```python
from build123d import *

# Parameters (mm, degrees)
F3_DEPTH  = 7.001
F4_W      = 1.95
F4_H      = 0.5
F5_DEPTH  = 4.75
F8_W      = 0.7
F8_H      = 0.5
F9_DEPTH  = 13.0048
F10_W     = 0.7
F10_H     = 0.5
F11_DEPTH = 10.9982


with BuildPart() as f1:
    # F0 (on Front) → F1 (revolve)
    with BuildSketch(Plane.XZ):
        with BuildLine():
            Line((-4.5, 0), (0, 0))
            Line((0, 0), (0, 7))
            ThreePointArc((0, 7), (-2.096194, 6.67877), (-4, 5.744563))
            Line((-4, 5.744563), (-4, 1.5))
            Line((-4, 1.5), (-4.5, 1.5))
            Line((-4.5, 1.5), (-4.5, 0))
        make_face()
    revolve(axis=Axis((0, 0, 3.5), (0, 0, 1)))

    # F2 (on face) → F3 (cut, through all)
    with BuildSketch(Plane(origin=(0, 0, 0), x_dir=(1, 0, 0), z_dir=(0, 0, -1))):
        with BuildLine():
            ThreePointArc((4, -2.061553), (4.5, 0), (4, 2.061553))
            Line((4, 2.061553), (4, -2.061553))
        make_face()
    extrude(amount=-F3_DEPTH, mode=Mode.SUBTRACT)

    # F4 (on face) → F5 (join)
    with BuildSketch(Plane(origin=(0, 0, 0), x_dir=(1, 0, 0), z_dir=(0, 0, -1))):
        with Locations((2.525, 0)):
            Rectangle(F4_W, F4_H)
        with Locations((-2.525, 0)):
            Rectangle(F4_W, F4_H)
    extrude(amount=F5_DEPTH)

    # F8 (on Front) → F9 (join)
    with BuildSketch(Plane.XZ):
        with Locations((-2.55, -5)):
            Rectangle(F8_W, F8_H)
    extrude(amount=F9_DEPTH)

    # F10 (on Front) → F11 (join)
    with BuildSketch(Plane.XZ):
        with Locations((2.55, -5)):
            Rectangle(F10_W, F10_H)
    extrude(amount=-F11_DEPTH)


solid = f1.part
```
Verification items for the finished model (mm, model axes). A direction names the side the tool comes from. Give positions to 0.01 mm unless a question says otherwise; leave off trailing zeros. Write each loop counter-clockwise with the first axis right and the second up, starting at its lowest first coordinate (ties: lowest second). Pieces come first, ordered by that corner, then holes. Notation, with made-up numbers: M 13.25,5 L 71.25,5 A16 cw 71.25,32 Z; hole C 34,40 d8. An arc over 180 degrees is marked long. One line per question, with ' | ' between items.
1) Thickness scan on line 1 along Y through (x, z) = (2.75, 3.75); line 2 along Y through (x, z) = (-2.5, -2); line 3 along Z through (x, y) = (-2.25, -0.5). Record the ranges inside material, lowest first. Write a range as [from, to].
Result:
line 1: y = [-2.9, 2.9] | line 2: y = [-0.25, 0.25] | line 3: z = [-5.25, -4.75], [0, 6.61]
2) Gauge pin test, flat ends, axial feed: pin 1 Ø2 at (x, z) = (2.5, -2.5) entering from +Y; pin 2 Ø1.6 at (x, z) = (2.5, -3.5) entering from -Y; pin 3 Ø1.5 at (x, y) = (1.5, 8) entering from +Z. Record the tip position at first contact, or that the pin passes through.
Result:
pin 1: stops at y = 0.25 | pin 2: stops at y = -0.25 | pin 3: stops at z = -4.75
3) Set-up check for faces 4 (the flat face through (3, -0.25, -2)), 5 (the flat face through (-3, 0.25, -2)), 6 (the cylindrical face through (0.867, 3.905, 3.593)): record each of +Z, -Z, +X, -X, +Y, -Y from which the full face is reachable in a straight line by a thin tool's end or side.
Result:
face 4: -Z, +X, -X, -Y | face 5: -Z, +X, -X, +Y | face 6: +Z
4) Mould release check, pull along Z, two halves, no side actions. Record for faces 1 (the flat face through (3, 0.25, -2)), 2 (the flat face through (4, 0, 1)), 3 (the flat face through (-3, -0.25, -2)): released by +Z, released by -Z, zero draft, split by the parting line, or undercut.
Result:
face 1: undercut | face 2: zero draft | face 3: undercut
5) Section check C-C on z = 4.25. Enter the section's corners in (x, y).
Result:
outline: C 0,0 d8
6) Section check A-A on z = -0.5. Enter the section's corners in (x, y).
Result:
outline: M -3.5,-0.25 L -1.55,-0.25 L -1.55,0.25 L -3.5,0.25 Z; M 1.55,-0.25 L 3.5,-0.25 L 3.5,0.25 L 1.55,0.25 Z
7) Section check B-B on y = -6.25. Enter the section's corners in (x, z), plus the area to 3 significant figures.
Result:
outline: M -2.9,-5.25 L -2.2,-5.25 L -2.2,-4.75 L -2.9,-4.75 Z | area: 0.350 mm2
